Check sheet for the drawn part. Datum: minimum x, y, z corner. Units: mm. Coordinates: 2 decimals unless noted, no trailing zeros. Write each loop counter-clockwise with the first axis right and the second up, starting at its lowest first coordinate (ties: lowest second). Pieces come first, ordered by that corner, then holes. Notation, with made-up numbers: M 77.25,9.5 L 86.25,9.5 A23 ccw 86.25,25.5 Z; hole C 61.25,79 d11. An arc over 180 degrees is marked long. Answer as CSV lines item,"result". Start each with the question number.
Q1. Sectioned sample at B-B, the plane z = 0.65. Record the cut outline in (x, y).
Q2. Thickness scan on line 1 along Y through (x, z) = (8, 0.6); line 2 along Y through (x, z) = (3, 1.05); line 3 along X through (y, z) = (3.5, 0.6). Record the ranges inside material, lowest first. Write a range as from..to.
Q3. Depth check by flat-ended pin: pin 1 Ø1.4 at (x, y) = (8, 4) entering from -Z. Enter the tip coordinate at first touch or a pass-through.
Q4. Sectioned sample at A-A, the plane x = 24. Record the cut outline in (y, z), then the cut area to 3 significant figures.
Q5. Sectioned sample at C-C, the plane x = 3. Record the cut outline in (y, z), then the cut area to 3 significant figures.
Q6. Sectioned sample at D-D, the plane y = 0.75. Record the cut outline in (x, z).
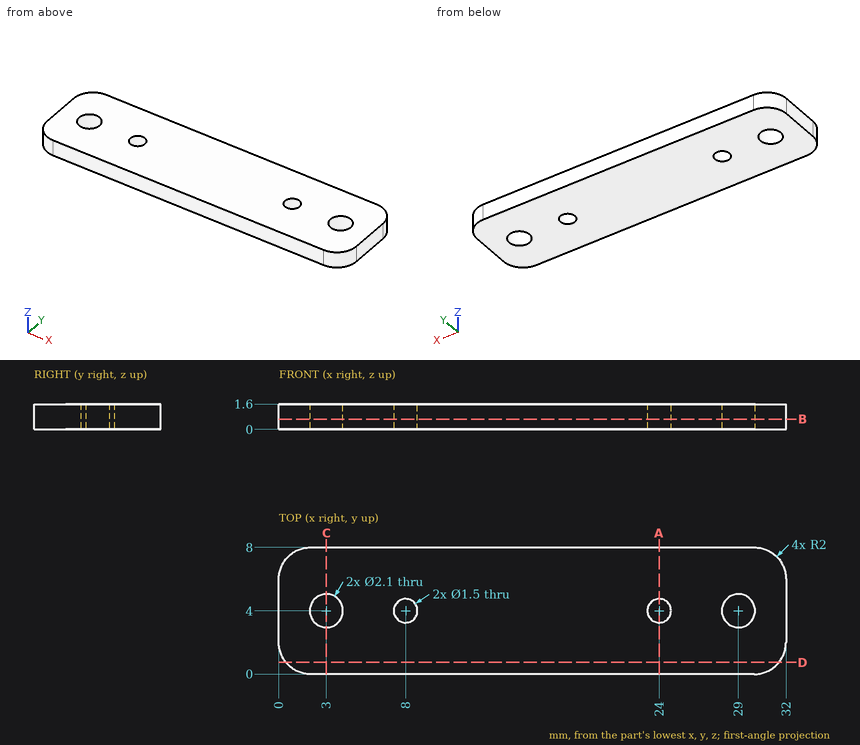
Output:
1,outline,"M 0,2 A2 ccw 2,0 L 30,0 A2 ccw 32,2 L 32,6 A2 ccw 30,8 L 2,8 A2 ccw 0,6 Z; hole C 3,4 d2.1; hole C 8,4 d1.5; hole C 24,4 d1.5; hole C 29,4 d2.1"
2,line 1,"y = 0..3.25, 4.75..8"
2,line 2,"y = 0..2.95, 5.05..8"
2,line 3,"x = 0..2.08, 3.92..7.44, 8.56..23.44, 24.56..28.08, 29.92..32"
3,pin 1,"passes through"
4,outline,"M 0,0 L 3.25,0 L 3.25,1.6 L 0,1.6 Z; M 4.75,0 L 8,0 L 8,1.6 L 4.75,1.6 Z"
4,area,"10.4 mm^2"
5,outline,"M 0,0 L 2.95,0 L 2.95,1.6 L 0,1.6 Z; M 5.05,0 L 8,0 L 8,1.6 L 5.05,1.6 Z"
5,area,"9.44 mm^2"
6,outline,"M 0.44,0 L 31.56,0 L 31.56,1.6 L 0.44,1.6 Z"
